Part model, mm, in its own coordinate system. A direction names the side the tool comes from. Give positions to 0.01 mm unless a question says otherwise; leave off trailing zeros. Order: outer loops, then holes, each group sorted by start corner. A loop starts at its lowest first (then second) coordinate and runs counter-clockwise, first axis right, second up. Notation, with made-up numbers: M 76,40.25 L 107,40.25 A23 cw 107,66.25 Z; hole C 46.5,76 d5. An arc over 180 degrees is marked long. Answer as a JSON object with one key per item and string values.
Autodesk Inventor part; units mm, degrees
ref_plane "Work Plane2" through (11.866, 9.4714, 3.25) normal (0.9239, 0.3827, 0) x (-0.3827, 0.9239, 0)
ref_plane "YZ Plane" through (0, 0, 0) normal (1, 0, 0) x (0, 1, 0)
ref_plane "XZ Plane" through (0, 0, 0) normal (0, 1, 0) x (-1, 0, 0)
sketch "Sketch1" plane through (0, 0, 0) normal (0, 0, 1) x (1, 0, 0)
  arc A0 (11, 0) -> (-11, 0) centre (0, 0) ccw
  arc A1 (14.0712, 3.5) -> (-14.0712, 3.5) centre (0, 0) ccw
  line L0 (-11, 0) -> (-18.5, 0)
  line L1 (-18.5, 0) -> (-18.5, 3.5)
  line L2 (11, 0) -> (18.5, 0)
  line L3 (18.5, 0) -> (18.5, 3.5)
  line L4 (-18.5, 3.5) -> (-14.0712, 3.5)
  line L5 (18.5, 3.5) -> (14.0712, 3.5)
  line L6 (-3.5, 15.0712) -> (3.5, 15.0712)
  line L7 (3.5, 15.0712) -> (3.5, 14.0712)
  line L8 (-3.5, 15.0712) -> (-3.5, 14.0712)
  point P0 (0, 15.0712)
  dimension "d2" = 11
  dimension "d3" = 14.5
  dimension "d4" = 7.5
  dimension "d5" = 3.5
  dimension "d6" = 18.5
  dimension "d7" = 7
  dimension "d8" = 1
extrude "Extrusion1" add sketch "Sketch1" along normal blind 6.5
sketch "Sketch2" plane through (0, 0, 6.5) normal (0, 0, 1) x (1, 0, 0)
  line L0 (-18.5, 3.5) -> (-18.5, 0)
  line L1 (-18.5, 0) -> (-11, 0)
  arc A0 (11, 0) -> (-11, 0) centre (0, 0) ccw
  line L2 (11, 0) -> (18.5, 0)
  line L3 (18.5, 0) -> (18.5, 3.5)
  line L4 (18.5, 3.5) -> (14.0712, 3.5)
  arc A1 (14.0712, 3.5) -> (3.5, 14.0712) centre (0, 0) ccw
  line L5 (3.5, 14.0712) -> (3.5, 15.0712)
  line L6 (3.5, 15.0712) -> (-3.5, 15.0712)
  line L7 (-3.5, 15.0712) -> (-3.5, 14.0712)
  arc A2 (-3.5, 14.0712) -> (-14.0712, 3.5) centre (0, 0) ccw
  line L8 (-14.0712, 3.5) -> (-18.5, 3.5)
  line L9 (0, 0) -> (18.5, 0)
  line L10 (0, 0) -> (23.4857, 9.7281)
  dimension "d11" = 22.5
ref_plane "Work Plane2" through (11.866, 9.4714, 3.25) normal (0.9239, 0.3827, 0) x (-0.3827, 0.9239, 0)
ref_plane "Work Plane1" through (-11, 0, 3.25) normal (0.9239, 0.3827, 0) x (-0.3827, 0.9239, 0)
sketch "Sketch3" plane through (11.866, 9.4714, 3.25) normal (0.9239, 0.3827, 0) x (-0.3827, 0.9239, 0)
  line L0 (-4.2095, 3.25) -> (-11.2892, 3.25)
  line L1 (-6.3608, -3.25) -> (7.4512, -3.25)
  line L2 (7.4512, -3.25) -> (7.4512, 3.25)
  line L3 (-6.3608, 3.25) -> (7.4512, 3.25)
  line L4 (-6.3608, -3.25) -> (-6.3608, 3.25)
  line L5 (-11.2892, -3.25) -> (-8.0556, -3.25)
  line L6 (-8.0556, -3.25) -> (-8.0556, 3.25)
  line L7 (-11.2892, 3.25) -> (-8.0556, 3.25)
  line L8 (-11.2892, -3.25) -> (-11.2892, 3.25)
  line L9 (-8.0556, -3.25) -> (-6.3608, -3.25)
  line L10 (-6.3608, -3.25) -> (-6.3608, 3.25)
  line L11 (-8.0556, 3.25) -> (-6.3608, 3.25)
  line L12 (-8.0556, -3.25) -> (-8.0556, 3.25)
  point P0 (-4.2095, -3.25)
  point P1 (-4.2095, 0)
  point P2 (-4.2095, 3.25)
  dimension "d13" = 3.25
  dimension "d14" = 11.6608
hole "Hole1" at (13.4769, 5.5823, 3.25) direction (-0.9239, -0.3827, 0) diameter 2 end through all
sketch "Sketch4" plane through (-3.5, 15.0712, 0) normal (0, 1, 0) x (1, 0, 0)
  line L0 (7, 0) -> (0, 0)
  line L1 (-15, 0) -> (-15, -6.5)
  point P0 (3.5, 0)
  point P1 (3.5, -3.25)
  point P2 (-15, -3.25)
  dimension "d22" = 18.5
  dimension "d23" = 3.25
hole "Hole2" at (0, 15.0712, 3.25) direction (0, -1, 0) diameter 2.459 end through all
sketch "Sketch5" plane through (-18.5, 3.5, 0) normal (0, 1, 0) x (1, 0, 0)
  line L0 (4.4288, 0) -> (0, 0)
  line L1 (0, 0) -> (0, -6.5)
  line L2 (37, 0) -> (37, -6.5)
  line L3 (37, 0) -> (32.5712, 0)
  point P0 (18.5, 0)
  point P1 (2.5, -3.25)
  point P2 (34.5, -3.25)
  point P3 (0, -3.25)
  dimension "d31" = 2.5
  dimension "d32" = 2.5
  dimension "d33" = 3.25
  dimension "d34" = 3.25
hole "Hole3" at (-16, 3.5, 3.25) at (16, 3.5, 3.25) direction (0, -1, 0) diameter 1.567 end through all
properties part number "29 - Sheave Strap 1" material "Steel AISI 1020 107 HR"
1. Cut at A-A on x = -16. Give the cut face in (y, z).
Worked answers:
{"outline": "M 0,0 L 3.5,0 L 3.5,2.47 L 0,2.47 Z; M 0,4.03 L 3.5,4.03 L 3.5,6.5 L 0,6.5 Z"}
2. Cut at D-D on y = 12.75. Give the cut face in (x, z).
Worked answers:
{"outline": "M -6.91,0 L 6.91,0 L 6.91,6.5 L -6.91,6.5 Z; hole C 0,3.25 d2.46"}
3. Pin check, flat tips, straight feed: P1, Ø2, axis at x = -15.5, z = 2, coming from the +Y side; P2, Ø2, axis at x = 0, z = 3.25, coming from the -Y side; P3, Ø1, axis at y = 6, z = 4, coming from the -X side; P4, Ø0.5, axis at y = 14.5, z = 2, coming from the +X side. Stop position of each tip, or through.
Worked answers:
{"P1": "stops at y = 3.5", "P2": "passes through", "P3": "stops at x = -13.42", "P4": "stops at x = 3.5"}
4. Cut at C-C on z = 3.25. Give the cut face in (x, y), plus the area to 3 significant figures.
Worked answers:
{"outline": "M -18.5,0 L -16.78,0 L -16.78,3.5 L -18.5,3.5 Z; M -15.22,0 L -11,0 A11 cw -1.23,10.93 L -1.23,15.07 L -3.5,15.07 L -3.5,14.07 A14.5 ccw -14.07,3.5 L -15.22,3.5 Z; M 1.23,10.93 A11 cw 9.74,5.12 L 12.98,6.46 A14.5 ccw 3.5,14.07 L 3.5,15.07 L 1.23,15.07 Z; M 10.5,3.27 A11 cw 11,0 L 15.22,0 L 15.22,3.5 L 14.07,3.5 A14.5 ccw 13.75,4.61 Z; M 16.78,0 L 18.5,0 L 18.5,3.5 L 16.78,3.5 Z", "area": "146 mm^2"}
5. Cut at B-B on y = 9. Give the cut face in (x, z).
Worked answers:
{"outline": "M -11.37,0 L -6.32,0 L -6.32,6.5 L -11.37,6.5 Z; M 6.32,0 L 11.37,0 L 11.37,6.5 L 6.32,6.5 Z"}
6. Probe line 1 along Z through (x, y) = (-16, 1.7); line 2 along Z through (x, y) = (0, 12); line 3 along X through (y, z) = (14.2, 3.25). List the from-to ranges inside material, lowest first.
Worked answers:
{"line 1": "z = 0 to 2.47, 4.03 to 6.5", "line 2": "z = 0 to 2.02, 4.48 to 6.5", "line 3": "x = -3.5 to -1.23, 1.23 to 3.5"}
7. Which spindle directions (+Z, -Z, +X, -X, +Y, -Y) get a long thin tool onto all of the face, cutting with end or side? Do faces 1 (the flat face through (-17, 3.5, 3)), 2 (the flat face through (3.5, 14.6, 3.2)), 3 (the flat face through (18.5, 2, 3)). Say none if no direction does.
Worked answers:
{"face 1": "+Z, -Z, -X, +Y", "face 2": "+Z, -Z, +X, +Y", "face 3": "+Z, -Z, +X, +Y, -Y"}
8. Two-plate mould, pull along X, no slides. Class faces 4 (the flat face through (15, 0, 3)), 5 (the cylindrical face through (10.175, 10.33, 3.204)), 6 (the cylindrical face through (0.748, 12.972, 2.274)): +X half, -X half, draft (parallel to the pull), parting line (faces both ways), or undercut.
Worked answers:
{"face 4": "draft", "face 5": "+X half", "face 6": "undercut"}
